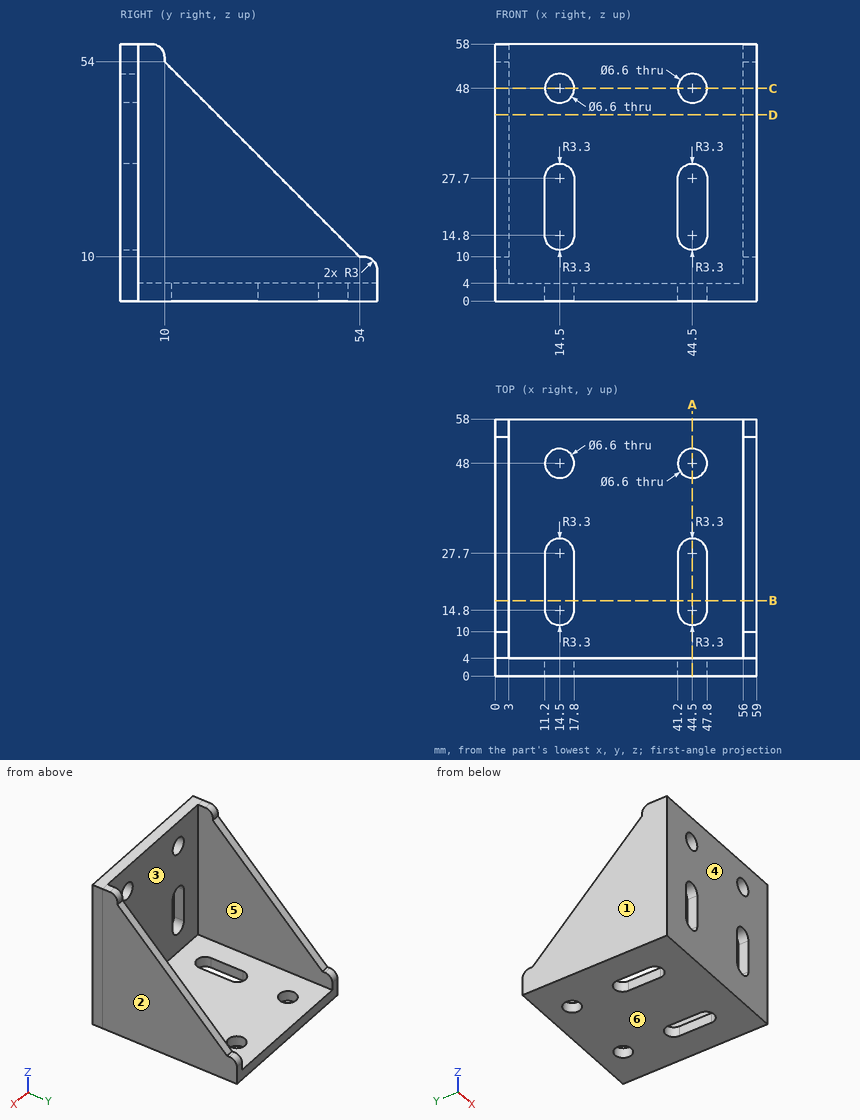
Could you check a few things on this drawing? It's one solid part, dimensions in mm from its lowest x, y, z. A direction names the side the tool comes from. Give positions to 0.01 mm unless a question says otherwise; leave off trailing zeros. Order: outer loops, then holes, each group sorted by start corner. A loop starts at its lowest first (then second) coordinate and runs counter-clockwise, first axis right, second up. Notation, with made-up numbers: (-10, 41) - (22, 41) arc R33 ccw to (22, 70) - close; hole circle Ø1 at (-36, 41.25). An arc over 180 degrees is marked (long way). One line per item, written item: value. Start each with the question number.
1. For the marked faces 5 and 6, which set-ups out of +Z, -Z, +X, -X, +Y, -Y let a thin tool reach every point of the face, with its end or its side?
2. Imagine slicing it at A-A on x = 44.5. List the corners of the cut face in (y, z) for me, plus the area to 3 significant figures.
3. Thinking about a two-plate mould opening in X: for the marked faces 1, 2, 3 and 4, which applies, +X half, -X half, draft (parallel to the pull), parting line (faces both ways), or undercut?
4. Imagine slicing it at B-B on y = 17. List the corners of the cut face in (x, z) for me.
5. Imagine slicing it at C-C on z = 48. List the corners of the cut face in (x, y) for me, plus the area to 3 significant figures.
6. For P1, Ø1.1, axis at x = 57, y = 54.5, coming from the +Z side; P2, Ø1.1, axis at x = 57, z = 54.5, coming from the +Y side; P3, Ø5, axis at x = 21.5, y = 17.5, coming from the +Z side; P4, Ø1, axis at y = 29.5, z = 36.5, coming from the -X side, each with a flat end and sliding along its axis, tell me the tip position at first contact or that it passes through.
7. Imagine slicing it at D-D on z = 42. List the corners of the cut face in (x, y) for me, plus the area to 3 significant figures.
8. If I drill on probe 1 along Y at (x, z) = (44.5, 1.95); probe 2 along X at (y, z) = (45, 11.5); probe 3 along Z at (x, y) = (33.5, 35.5), over which ranges is the centre line in solid material (lowest first)?
Values:
1. face 5: +Z, +Y
1. face 6: -Z, +X, -X, +Y, -Y
2. outline: (0, 0) - (11.5, 0) - (11.5, 4) - (4, 4) - (4, 11.5) - (0, 11.5) - close; (0, 31) - (4, 31) - (4, 44.7) - (0, 44.7) - close; (0, 51.3) - (4, 51.3) - (4, 58) - (0, 58) - close; (31, 0) - (44.7, 0) - (44.7, 4) - (31, 4) - close; (51.3, 0) - (58, 0) - (58, 4) - (51.3, 4) - close
2. area: 239 mm²
3. face 1: -X half
3. face 2: +X half
3. face 3: undercut
3. face 4: draft
4. outline: (0, 0) - (11.2, 0) - (11.2, 4) - (3, 4) - (3, 47) - (0, 47) - close; (17.8, 0) - (41.2, 0) - (41.2, 4) - (17.8, 4) - close; (47.8, 0) - (59, 0) - (59, 47) - (56, 47) - (56, 4) - (47.8, 4) - close
5. outline: (0, 0) - (11.2, 0) - (11.2, 4) - (3, 4) - (3, 16) - (0, 16) - close; (17.8, 0) - (41.2, 0) - (41.2, 4) - (17.8, 4) - close; (47.8, 0) - (59, 0) - (59, 16) - (56, 16) - (56, 4) - (47.8, 4) - close
5. area: 255 mm²
6. P1: z = 10.05
6. P2: y = 10.05
6. P3: z = 4
6. P4: through
7. outline: (0, 0) - (59, 0) - (59, 22) - (56, 22) - (56, 4) - (3, 4) - (3, 22) - (0, 22) - close
7. area: 344 mm²
8. probe 1: 0 to 11.5, 31 to 44.7, 51.3 to 58
8. probe 2: 0 to 3, 56 to 59
8. probe 3: 0 to 4
